For this review, use the dimensioned drawing (mm, ordinates from the lowest corner) and the shaded views. A direction names the side the tool comes from. Round coordinates to 2 decimals unless told otherwise and drop trailing zeros. Loops run counter-clockwise (first coordinate to the right, second up) from the corner with the lowest first, then second, coordinate; pieces in that order, holes last. Notation, with made-up numbers: M -37.75,62 L -20.75,62 A25 ccw -20.75,87 Z; hole C 63,72 d2. An arc over 180 degrees is marked long. One line per item, written item: value. Start each with the question number.
Item 1: We need section A-A (y = 8.5). Write out the cut boundary in (x, z) (1 decimal).
Item 2: We need section D-D (y = 4.25). Write out the cut boundary in (x, z) (1 decimal), then the cut area to 3 significant figures.
Item 3: For the marked faces 1, 2 and 3, list the 3-axis set-ups (+Z, -Z, +X, -X, +Y, -Y) from which the entire face can be reached by the end or side of a thin tool; tool diameter is ignored.
Item 4: Clearance check with flat-ended pins moving along their axes: pin 1 (4 mm diameter, centred on y = 12, z = 17.5, fed in from +X); pin 2 (1.5 mm diameter, centred on y = 10.5, z = 9, fed in from +X); pin 3 (4 mm diameter, centred on x = 9.59, z = 5, fed in from -Y) (3 decimals). State where each tip first meets the part, or that it passes through.
Item 5: We need section C-C (x = 8.75). Write out the cut boundary in (y, z), then the cut area to 3 significant figures.
Item 6: We need section B-B (z = 5.5). Write out the cut boundary in (x, y) (1 decimal).
Item 7: Mouldability with a two-part tool opening along Z and no side actions: class the marked faces 4, 5 and 6 as released by +Z, released by -Z, zero draft, split by the parting line, or undercut.
Item 8: For line 1 along Z through (x, y) = (6, 2.75); line 2 along X through (y, z) = (12.25, 19.5); line 3 along Z through (x, y) = (16.5, 3.5), list the stretches that pass through material, from the lowest coordinate up.
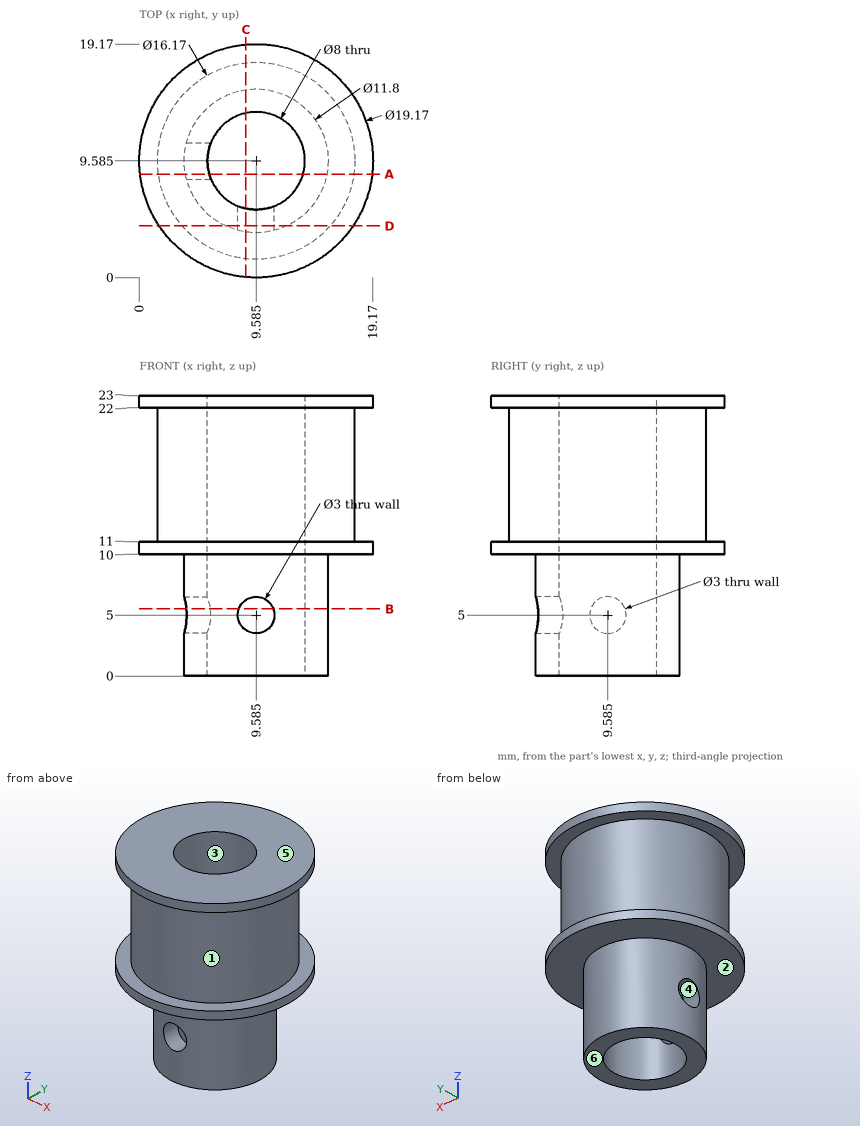
A:
1. outline: M 0.1,10 L 3.8,10 L 3.8,6 L 5.7,6 L 5.7,23 L 0.1,23 L 0.1,22 L 1.6,22 L 1.6,11 L 0.1,11 Z; M 3.8,0 L 5.7,0 L 5.7,4 L 3.8,4 Z; M 13.4,0 L 15.4,0 L 15.4,10 L 19.1,10 L 19.1,11 L 17.6,11 L 17.6,22 L 19.1,22 L 19.1,23 L 13.4,23 Z
2. outline: M 1.6,10 L 7.1,10 L 7.1,0 L 12.1,0 L 12.1,10 L 17.5,10 L 17.5,11 L 15.7,11 L 15.7,22 L 17.5,22 L 17.5,23 L 1.6,23 L 1.6,22 L 3.5,22 L 3.5,11 L 1.6,11 Z; hole C 9.6,5 d3
2. area: 209 mm2
3. face 1: none
3. face 2: -Z
3. face 3: +Z, -Z
4. pin 1: x = 17.66
4. pin 2: x = 15.48
4. pin 3: y = 3.685
5. outline: M 0.04,10 L 3.74,10 L 3.74,6.25 L 5.67,6.25 L 5.67,23 L 0.04,23 L 0.04,22 L 1.54,22 L 1.54,11 L 0.04,11 Z; M 3.74,0 L 5.67,0 L 5.67,3.75 L 3.74,3.75 Z; M 13.5,0 L 15.43,0 L 15.43,10 L 19.13,10 L 19.13,11 L 17.63,11 L 17.63,22 L 19.13,22 L 19.13,23 L 13.5,23 Z
5. area: 147 mm2
6. outline: M 3.9,8.2 A5.9 ccw 8.2,3.9 L 8.2,5.8 A4 cw 5.8,8.2 Z; M 3.9,11 L 5.8,11 A4 cw long 11,5.8 L 11,3.9 A5.9 ccw long Z
7. face 4: undercut
7. face 5: released by +Z
7. face 6: released by -Z
8. line 1: 10 to 23
8. line 2: 1.95 to 6.6, 12.57 to 17.22
8. line 3: 10 to 11, 22 to 23
